Could you check a few things on this model? Use its own coordinates, in mm. A direction names the side the tool comes from. Give positions to 0.01 mm unless a question says otherwise; leave off trailing zeros. Loops run counter-clockwise (first coordinate to the right, second up) from the corner with the lowest first, then second, coordinate; pieces in that order, holes last. Notation, with made-up numbers: M 82.25,34.25 L 110.25,34.25 A22 ccw 110.25,58.25 Z; hole C 4.5,-6.75 d1. An arc over 180 degrees is marked long. Use a Markdown table: item, result. Add a question column.
1) Suppose I cut it at A-A on z = 4.5. List the corners of the cut face in (x, y) for me.
2) Suppose I cut it at D-D on y = -3. List the corners of the cut face in (x, z) for me.
3) We'd pull the mould along X, two halves only. Please class faces 5 (the cylindrical face through (-1.5, -2.43, 4.43)), 6 (the flat face through (-0.5, -1, -5)), 7 (the flat face through (-1, -1, -1)): +X half, -X half, draft (parallel to the pull), parting line (faces both ways), or undercut.
4) Suppose I cut it at B-B on x = -1. List the corners of the cut face in (y, z) for me, and give its area (3 significant figures).
5) Suppose I cut it at C-C on z = -4. List the corners of the cut face in (x, y) for me, and give its area (3 significant figures).
6) Which directions (+Z, -Z, +X, -X, +Y, -Y) give clear straight access to the entire face, cutting with the end or side of a thin tool? Please do faces 1 (the flat face through (0.5, 1, -5)), 2 (the cylindrical face through (0, 2.5, -5.4)), 3 (the flat face through (-1, -0.5, -5)), 4 (the cylindrical face through (0, -2.5, -5.4)).
7) Will these pins go through, and if not, where does the flat tip stop? pin 1 Ø1.6 at (x, z) = (1.5, -4.5) entering from +Y; pin 2 Ø1.8 at (x, y) = (-0.5, 0.5) entering from +Z; pin 3 Ø1.3 at (x, y) = (1, 1) entering from +Z; pin 4 Ø1 at (x, z) = (-1.5, 0) entering from -Y.
8) If I drill on line 1 along Z through (x, y) = (0, -2.85); line 2 along Y through (x, z) = (0, 7); line 3 along X through (y, z) = (-2.5, 3.25), over which ranges is the centre line in solid material (lowest first)? Write a range as [from, to].
```python
from build123d import *

# Parameters (mm, degrees)
SKETCH1_R               = 4
SKETCH1_R_2             = 1.75
BOSS_EXTRUDE1_DEPTH     = 10
SKETCH2_W               = 1
SKETCH2_H               = 1
BOSS_EXTRUDE2_DEPTH     = 10
SKETCH3_R               = 4
BOSS_EXTRUDE3_DEPTH     = 1
SKETCH4_R               = 1.5
CUT_EXTRUDE1_DEPTH      = 5
CUT_EXTRUDE1_DEPTH_BACK = 5


with BuildPart() as part:
    # Sketch1 → Boss-Extrude1 (new body)
    with BuildSketch(Plane.XY):
        Circle(SKETCH1_R)
        Circle(SKETCH1_R_2, mode=Mode.SUBTRACT)
    extrude(amount=BOSS_EXTRUDE1_DEPTH)

    # Sketch2 → Boss-Extrude2 (add)
    with BuildSketch(Plane(origin=(0, 0, 0), x_dir=(-1, 0, 0), z_dir=(0, 0, -1))):
        with BuildLine():
            ThreePointArc((0.5, 1.677050983), (0, 1.75), (-0.5, 1.677050983))
            Line((-0.5, 1.677050983), (-0.5, 0.5))
            Line((-0.5, 0.5), (0.5, 0.5))
            Line((0.5, 0.5), (0.5, 1.677050983))
        make_face()
        with BuildLine():
            ThreePointArc((0.5, 2.449489743), (0, 2.5), (-0.5, 2.449489743))
            Line((-0.5, 2.449489743), (-0.5, 1.677050983))
            ThreePointArc((-0.5, 1.677050983), (0, 1.75), (0.5, 1.677050983))
            Line((0.5, 1.677050983), (0.5, 2.449489743))
        make_face()
        with BuildLine():
            Line((-0.5, -1.677050983), (-0.5, -2.449489743))
            ThreePointArc((-0.5, -2.449489743), (0, -2.5), (0.5, -2.449489743))
            Line((0.5, -2.449489743), (0.5, -1.677050983))
            ThreePointArc((0.5, -1.677050983), (0, -1.75), (-0.5, -1.677050983))
        make_face()
        with BuildLine():
            Line((-0.5, -0.5), (-0.5, 0.5))
            Line((-0.5, 0.5), (-1.677050983, 0.5))
            ThreePointArc((-1.677050983, 0.5), (-1.75, 0), (-1.677050983, -0.5))
            Line((-1.677050983, -0.5), (-0.5, -0.5))
        make_face()
        with BuildLine():
            Line((-1.677050983, 0.5), (-2.449489743, 0.5))
            ThreePointArc((-2.449489743, 0.5), (-2.5, 0), (-2.449489743, -0.5))
            Line((-2.449489743, -0.5), (-1.677050983, -0.5))
            ThreePointArc((-1.677050983, -0.5), (-1.75, 0), (-1.677050983, 0.5))
        make_face()
        with BuildLine():
            ThreePointArc((2.5, 0), (2.487340383, 0.251272405), (2.449489743, 0.5))
            Line((2.449489743, 0.5), (1.677050983, 0.5))
            ThreePointArc((1.677050983, 0.5), (1.731666715, 0.252646769), (1.75, 0))
            ThreePointArc((1.75, 0), (1.731666715, -0.252646769), (1.677050983, -0.5))
            Line((1.677050983, -0.5), (2.449489743, -0.5))
            ThreePointArc((2.449489743, -0.5), (2.487340383, -0.251272405), (2.5, 0))
        make_face()
        with BuildLine():
            Line((0.5, -0.5), (-0.5, -0.5))
            Line((-0.5, -0.5), (-0.5, -1.677050983))
            ThreePointArc((-0.5, -1.677050983), (0, -1.75), (0.5, -1.677050983))
            Line((0.5, -1.677050983), (0.5, -0.5))
        make_face()
        Rectangle(SKETCH2_W, SKETCH2_H)
        with BuildLine():
            Line((1.677050983, 0.5), (0.5, 0.5))
            Line((0.5, 0.5), (0.5, -0.5))
            Line((0.5, -0.5), (1.677050983, -0.5))
            ThreePointArc((1.677050983, -0.5), (1.731666715, -0.252646769), (1.75, 0))
            ThreePointArc((1.75, 0), (1.731666715, 0.252646769), (1.677050983, 0.5))
        make_face()
    extrude(amount=BOSS_EXTRUDE2_DEPTH)

    # Sketch3 → Boss-Extrude3 (add)
    with BuildSketch(Plane(origin=(0, 0, 0), x_dir=(-1, 0, 0), z_dir=(0, 0, -1))):
        Circle(SKETCH3_R)
    extrude(amount=BOSS_EXTRUDE3_DEPTH)

    # Sketch4 → Cut-Extrude1 (cut, two sides)
    with BuildSketch(Plane(origin=(0, 0, 0), x_dir=(1, 0, 0), z_dir=(0, 1, 0))) as cut_extrude1_sk:
        with Locations((0, -4.5)):
            Circle(SKETCH4_R)
    extrude(amount=CUT_EXTRUDE1_DEPTH, mode=Mode.SUBTRACT)
    extrude(cut_extrude1_sk.sketch, amount=-CUT_EXTRUDE1_DEPTH_BACK, mode=Mode.SUBTRACT)


solid = part.part
```
Answer block:
| question | item | result |
|---|---|---|
| 1 | outline | M -1.5,-3.71 L -1.5,-0.9 A1.75 cw -1.5,0.9 L -1.5,3.71 A4 ccw Z; M 1.5,-3.71 A4 ccw 1.5,3.71 L 1.5,0.9 A1.75 cw 1.5,-0.9 Z |
| 2 | outline | M -2.65,-1 L 2.65,-1 L 2.65,10 L -2.65,10 Z; hole C 0,4.5 d3 |
| 3 | face 5 | undercut |
| 3 | face 6 | -X half |
| 3 | face 7 | draft |
| 4 | outline | M -3.87,-1 L -0.5,-1 L -0.5,-10 L 0.5,-10 L 0.5,-1 L 3.87,-1 L 3.87,3.38 L 1.44,3.38 L 1.44,0 L -1.44,0 L -1.44,3.38 L -3.87,3.38 Z; M -3.87,5.62 L -1.44,5.62 L -1.44,10 L -3.87,10 Z; M 1.44,5.62 L 3.87,5.62 L 3.87,10 L 1.44,10 Z |
| 4 | area | 54.6 mm^2 |
| 5 | outline | M -2.45,-0.5 L -0.5,-0.5 L -0.5,-2.45 A2.5 ccw 0.5,-2.45 L 0.5,-0.5 L 2.45,-0.5 A2.5 ccw 2.45,0.5 L 0.5,0.5 L 0.5,2.45 A2.5 ccw -0.5,2.45 L -0.5,0.5 L -2.45,0.5 A2.5 ccw Z |
| 5 | area | 8.93 mm^2 |
| 6 | face 1 | -Z, +X, +Y |
| 6 | face 2 | -Z, +Y |
| 6 | face 3 | -Z, -X, -Y |
| 6 | face 4 | -Z, -Y |
| 7 | pin 1 | stops at y = 0.5 |
| 7 | pin 2 | stops at z = 0 |
| 7 | pin 3 | stops at z = 10 |
| 7 | pin 4 | stops at y = -3.87 |
| 8 | line 1 | z = [-1, 3], [6, 10] |
| 8 | line 2 | y = [-4, -1.75], [1.75, 4] |
| 8 | line 3 | x = [-3.12, -0.83], [0.83, 3.12] |
